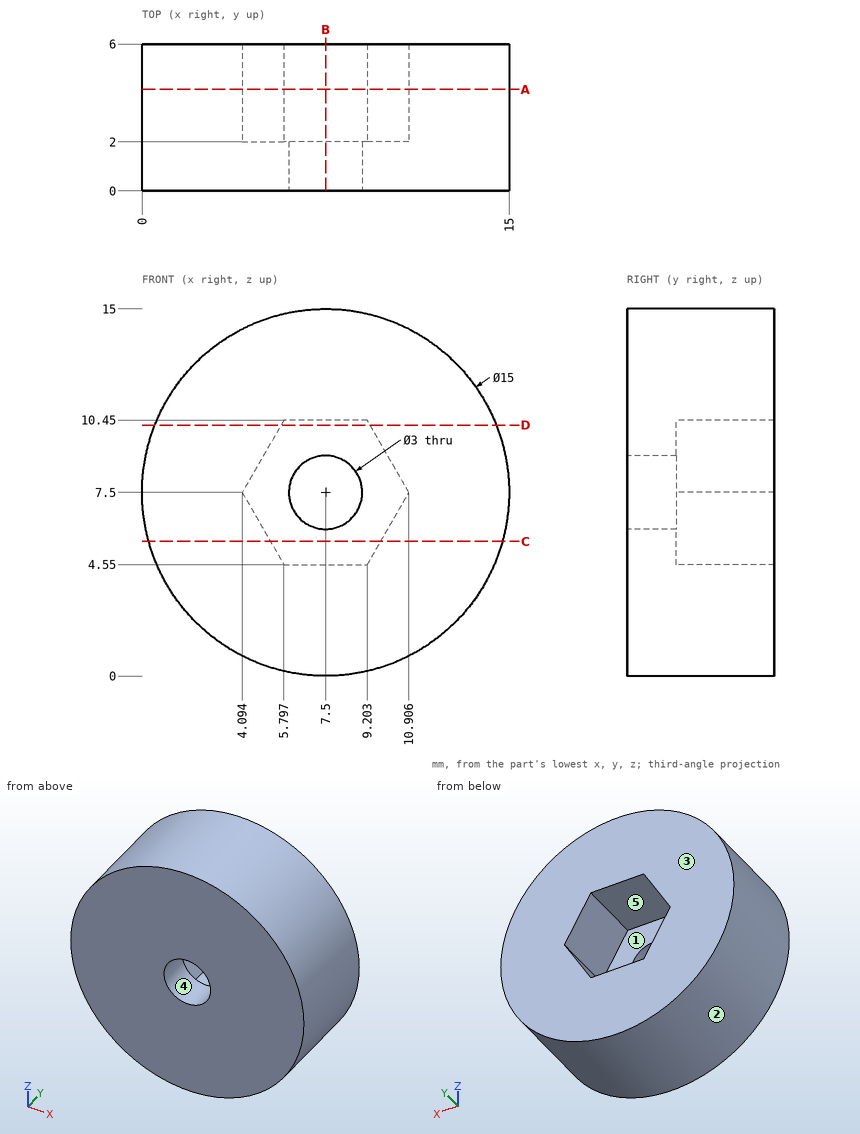
The figure shows three views and two pictorial views of one solid part (mm, origin at its lowest corner). Answer the questions. A direction names the side the tool comes from. Coordinates: 2 decimals unless noted, no trailing zeros. Order: outer loops, then holes, each group sorted by start corner. A loop starts at its lowest first (then second) coordinate and runs counter-clockwise, first axis right, second up.
Q1. Given P1, Ø3.5, axis at x = 8, y = 4, coming from the +Z side; P2, Ø1.5, axis at x = 2.5, y = 5, coming from the -Z side; P3, Ø1.5, axis at y = 4.5, z = 11, coming from the -X side; P4, Ø1.5, axis at x = 13.5, y = 2.5, coming from the -Z side (1 decimal), each flat-ended and moving along its own axis, determine where each tip first touches the part or whether it passes through.
Q2. A cutting plane is placed at B-B, the plane x = 7.5. Write down the section's boundary in (y, z), and give its area (3 significant figures).
Q3. Consider line 1 (Z direction, x = 7.5, y = 0.4); line 2 (Z direction, x = 10, y = 3.4); line 3 (Y direction, x = 6.5, z = 9). Determine where each line is inside the solid, lowest interval first.
Q4. A cutting plane is placed at A-A, the plane y = 4.15. Write down the section's boundary in (x, z), and give its area (3 significant figures).
Q5. A cutting plane is placed at C-C, the plane z = 5.5. Write down the section's boundary in (x, y).
Q6. A cutting plane is placed at D-D, the plane z = 10.25. Write down the section's boundary in (x, y).
Q7. Which of the six approach directions +Z, -Z, +X, -X, +Y, -Y give full straight-line access (tool end or side, diameter ignored) to the marked faces 4 and 5?
Q8. For a pull along X with two mould halves and no side action, classify the marked faces 1, 2 and 3 as pulls with the +X half, pulls with the -X half, needs draft (parallel to the pull), parting line crosses it, or undercut.
Answers follow:
1. P1: stops at z = 15
1. P2: stops at z = 1.32
1. P3: stops at x = 0.52
1. P4: stops at z = 2.1
2. outline: (0, 0) - (6, 0) - (6, 4.55) - (2, 4.55) - (2, 6) - (0, 6) - close; (0, 9) - (2, 9) - (2, 10.45) - (6, 10.45) - (6, 15) - (0, 15) - close
2. area: 60.4 mm2
3. line 1: z = 0 to 6, 9 to 15
3. line 2: z = 0.43 to 5.93, 9.07 to 14.57
3. line 3: y = 0 to 2
4. outline: circle Ø15 at (7.5, 7.5); hole (4.09, 7.5) - (5.8, 4.55) - (9.2, 4.55) - (10.91, 7.5) - (9.2, 10.45) - (5.8, 10.45) - close
4. area: 147 mm2
5. outline: (0.27, 0) - (14.73, 0) - (14.73, 6) - (9.75, 6) - (9.75, 2) - (5.25, 2) - (5.25, 6) - (0.27, 6) - close
6. outline: (0.52, 0) - (14.48, 0) - (14.48, 6) - (9.32, 6) - (9.32, 2) - (5.68, 2) - (5.68, 6) - (0.52, 6) - close
7. face 4: +Y, -Y
7. face 5: +Y
8. face 1: undercut
8. face 2: parting line crosses it
8. face 3: needs draft
